Design review of the part shown in the three views and the two pictorial views. Dimensions are in mm from the part's minimum x, y and z. A direction names the side the tool comes from. Round coordinates to 2 decimals unless told otherwise and drop trailing zeros. Order: outer loops, then holes, each group sorted by start corner. A loop starts at its lowest first (then second) coordinate and runs counter-clockwise, first axis right, second up. Notation, with made-up numbers: (42, 13.5) - (63, 13.5) arc R32 ccw to (63, 45.5) - close; hole circle Ø2 at (-24.75, 56). An arc over 180 degrees is marked (long way). One line per item, written item: value.
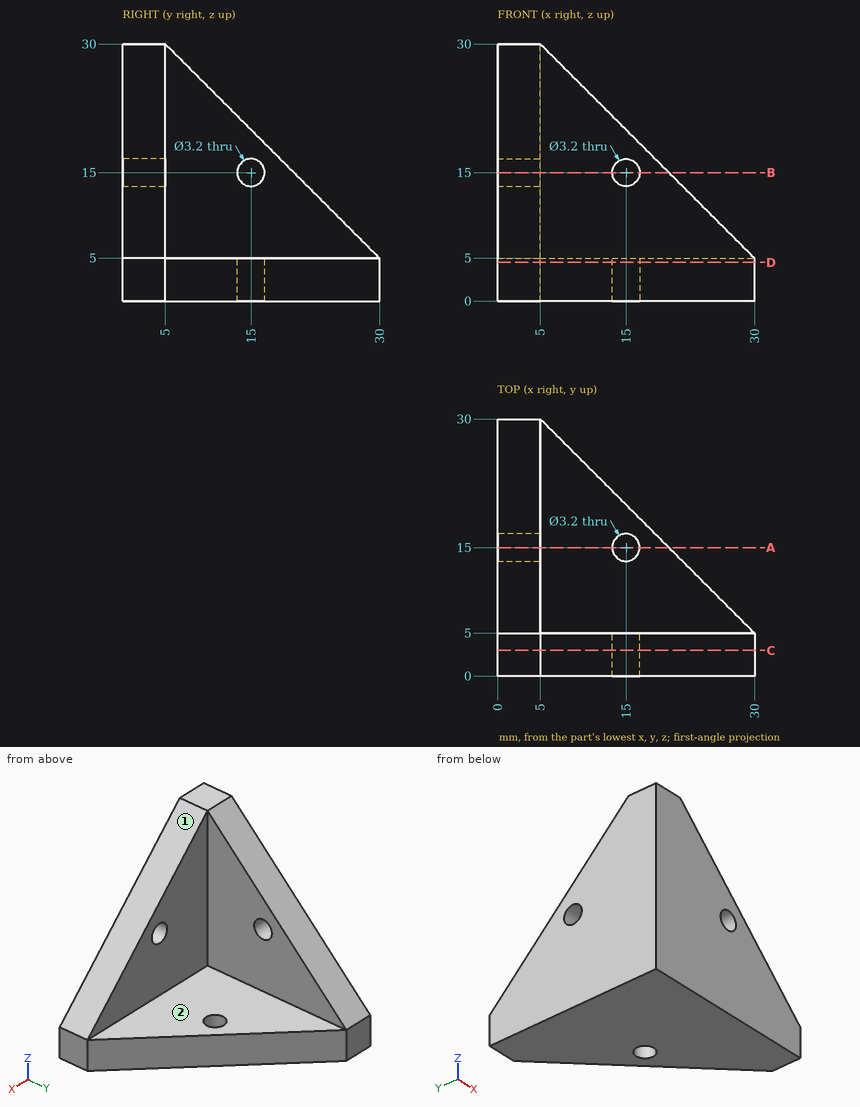
Item 1: For P1, Ø5, axis at x = 22.5, z = 13.5, coming from the +Y side; P2, Ø1.5, axis at y = 11, z = 8.5, coming from the -X side; P3, Ø7.5, axis at x = 12.5, y = 21, coming from the +Z side; P4, Ø10, axis at y = 10.5, z = 24, coming from the +X side, all flat-tipped, find the tip position at first contact; note any pin that passes through.
Returned:
P1: y = 5
P2: x = 0
P3: z = 5
P4: x = 5
Item 2: Wall thickness on line 1 (Z direction, x = 3.3, y = 15); line 2 (Y direction, x = 20.5, z = 10.5): over which ranges is each line inside the solid? List them lowest first.
Returned:
line 1: 0 to 13.4, 16.6 to 20
line 2: 0 to 5
Item 3: Machinability: for the marked faces 1 and 2, which of the approach directions +Z, -Z, +X, -X, +Y, -Y give a long, thin tool a straight path to every point of the face, cutting with its end or side? Answer none if there is none.
Returned:
face 1: +Z, +X, +Y, -Y
face 2: +Z, +X, +Y
Item 4: Take a section at A-A (y = 15). Write out the cut boundary in (x, z).
Returned:
outline: (0, 0) - (13.4, 0) - (13.4, 5) - (5, 5) - (5, 13.4) - (0, 13.4) - close; (0, 16.6) - (5, 16.6) - (5, 20) - (0, 20) - close; (16.6, 0) - (20, 0) - (20, 5) - (16.6, 5) - close
Item 5: Take a section at C-C (y = 3). Write out the cut boundary in (x, z), plus the area to 3 significant figures.
Returned:
outline: (0, 0) - (30, 0) - (30, 5) - (5, 30) - (0, 30) - close; hole circle Ø3.2 at (15, 15)
area: 579 mm^2
